Geometry check sheet. Reference: drawing and pictorial views, mm from the part's lowest x, y, z. A direction names the side the tool comes from. Give positions to 0.01 mm unless a question says otherwise; leave off trailing zeros. Order: outer loops, then holes, each group sorted by start corner. A loop starts at its lowest first (then second) coordinate and runs counter-clockwise, first axis right, second up. Notation, with made-up numbers: (9.5, 89.25) -> (17.5, 89.25) arc R13 cw to (17.5, 107.25) -> close; hole circle Ø6 at (30, 20). An arc over 180 degrees is marked (long way). Write each question's results on one line, items separated by ' | '. Start each with the question number.
1. Cross-section at B-B, the plane z = 12.7. Enter the section's corners in (x, y) (3 decimals).
2. Material ranges on L1, parallel to Y at x = 12.7, z = 48.8 (3 decimals); L2, parallel to Z at x = 12, y = 1; L3, parallel to Z at x = 15.5, y = 13.5 (3 decimals), recorded low to high. Write a range as from..to.
3. Set-up check for the marked faces 1 and 2: record each of +Z, -Z, +X, -X, +Y, -Y from which the full face is reachable in a straight line by a thin tool's end or side.
4. Depth check by flat-ended pin: pin 1 Ø4.5 at (x, z) = (12.7, 12.7) entering from -Y; pin 2 Ø20.5 at (x, y) = (16, 26) entering from -Z (3 decimals); pin 3 Ø10 at (x, z) = (31.5, 31) entering from +Y (3 decimals); pin 4 Ø1.5 at (x, y) = (25, 8) entering from -Z. Enter the tip coordinate at first touch or a pass-through.
5. Cross-section at D-D, the plane x = 27. Enter the section's corners in (y, z) (3 decimals), then the cut area to 3 significant figures.
6. Cross-section at C-C, the plane y = 38.1. Enter the section's corners in (x, z) (3 decimals).
7. Cross-section at A-A, the plane x = 38.1. Enter the section's corners in (y, z) (3 decimals), then the cut area to 3 significant figures.
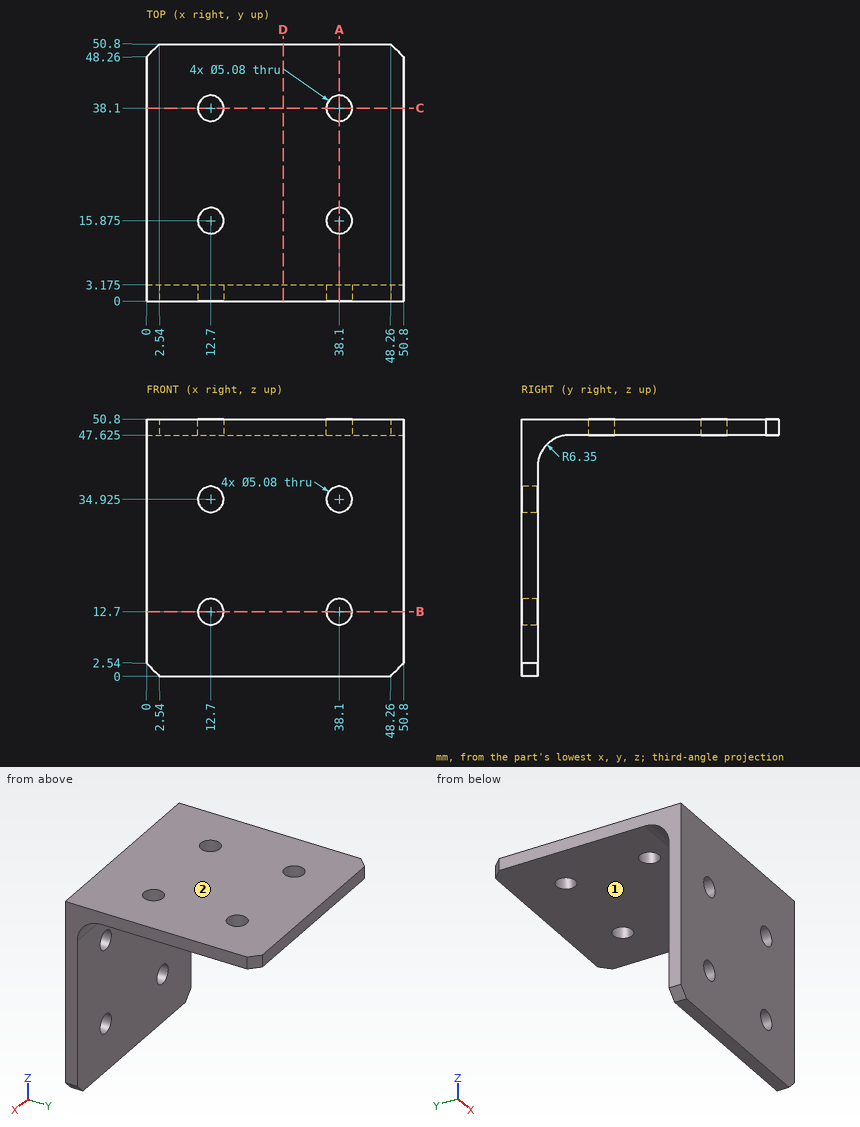
Results below:
1) outline: (0, 0) -> (10.16, 0) -> (10.16, 3.175) -> (0, 3.175) -> close; (15.24, 0) -> (35.56, 0) -> (35.56, 3.175) -> (15.24, 3.175) -> close; (40.64, 0) -> (50.8, 0) -> (50.8, 3.175) -> (40.64, 3.175) -> close
2) L1: y = 0..13.335, 18.415..35.56, 40.64..50.8 | L2: z = 0..10.26, 15.14..32.48, 37.37..50.8 | L3: z = 47.625..50.8
3) face 1: -Z, +X, -X, +Y | face 2: +Z, +X, -X, +Y, -Y
4) pin 1: passes through | pin 2: stops at z = 47.625 | pin 3: stops at y = 3.175 | pin 4: stops at z = 47.2
5) outline: (0, 0) -> (3.175, 0) -> (3.175, 41.275) arc R6.35 cw to (9.525, 47.625) -> (50.8, 47.625) -> (50.8, 50.8) -> (0, 50.8) -> close | area: 321 mm²
6) outline: (0, 47.625) -> (10.16, 47.625) -> (10.16, 50.8) -> (0, 50.8) -> close; (15.24, 47.625) -> (35.56, 47.625) -> (35.56, 50.8) -> (15.24, 50.8) -> close; (40.64, 47.625) -> (50.8, 47.625) -> (50.8, 50.8) -> (40.64, 50.8) -> close
7) outline: (0, 0) -> (3.175, 0) -> (3.175, 10.16) -> (0, 10.16) -> close; (0, 15.24) -> (3.175, 15.24) -> (3.175, 32.385) -> (0, 32.385) -> close; (0, 37.465) -> (3.175, 37.465) -> (3.175, 41.275) arc R6.35 cw to (9.525, 47.625) -> (13.335, 47.625) -> (13.335, 50.8) -> (0, 50.8) -> close; (18.415, 47.625) -> (35.56, 47.625) -> (35.56, 50.8) -> (18.415, 50.8) -> close; (40.64, 47.625) -> (50.8, 47.625) -> (50.8, 50.8) -> (40.64, 50.8) -> close | area: 257 mm²
